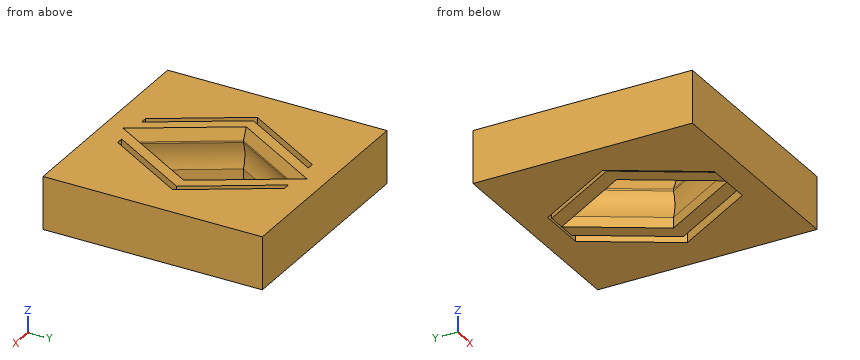
```python
from build123d import *

# Parameters (mm, degrees)
SKETCH_W      = 25
SKETCH_H      = 25
PAD_DEPTH     = 6
CHAMFER_SIZE2 = 1.3
CHAMFER_SIZE  = 0.5
POCKET_DEPTH  = 0.3


with BuildPart() as part:
    # Sketch (on XY_Plane of Origin) → Pad (new body)
    with BuildSketch(Plane.XY):
        Rectangle(SKETCH_W, SKETCH_H)
        Polygon((0, 9.5), (-5.7, 0), (0, -9.5), (5.7, 0), align=None, mode=Mode.SUBTRACT)
        Polygon((-2, 9.5), (-7.7, 0), (-2, -9.5), (-2.8, -9.5), (-8.5, 0), (-2.8, 9.5), align=None, mode=Mode.SUBTRACT)
        Polygon((2, -9.5), (7.7, 0), (2, 9.5), (2.8, 9.5), (8.5, 0), (2.8, -9.5), align=None, mode=Mode.SUBTRACT)
    extrude(amount=PAD_DEPTH)

    # Sketch002 (on Face22 of Pad) → SubtractiveLoft section 0
    with BuildSketch(Plane.XY.offset(4.5)):
        Polygon((-5.7, 0), (0, -9.5), (5.7, 0), (0, 9.5), align=None)
    # Sketch001 (on Face22 of Pad) → SubtractiveLoft section 1
    with BuildSketch(Plane.XY.offset(3)):
        Polygon((-6, 0), (0, 10), (6, 0), (0, -10), align=None)
    # Sketch003 (on Face22 of Pad) → SubtractiveLoft section 2
    with BuildSketch(Plane.XY.offset(1.5)):
        Polygon((-5.7, 0), (0, 9.5), (5.7, 0), (0, -9.5), align=None)
    loft(mode=Mode.SUBTRACT)

    # Chamfer
    chamfer_edges = [part.edges().sort_by_distance(p)[0] for p in [
        (2.85, 4.75, 6),
        (-2.85, 4.75, 6),
        (-2.85, -4.75, 6),
        (2.85, -4.75, 6),
    ]]
    chamfer_side = part.faces().sort_by_distance((-12.146447, 0, 6))[0]
    chamfer(chamfer_edges, length=CHAMFER_SIZE, length2=CHAMFER_SIZE2, reference=chamfer_side)

    # Sketch004 (on Face4 of SubtractiveLoft) → Pocket (cut)
    with BuildSketch(Plane(origin=(0, 0, 0), x_dir=(1, 0, 0), z_dir=(0, 0, -1))):
        Polygon((-8.5, 0), (-2.8, -9.5), (2.8, -9.5), (8.5, 0), (2.8, 9.5), (-2.8, 9.5), align=None)
    extrude(amount=-POCKET_DEPTH, mode=Mode.SUBTRACT)


solid = part.part
```
CAD build for the part. Positions are in the model's coordinates, mm. Round coordinates to 2 decimals unless told otherwise and drop trailing zeros. Loops run counter-clockwise (first coordinate to the right, second up) from the corner with the lowest first, then second, coordinate; pieces in that order, holes last. Notation, with made-up numbers: M 35.25,72.5 L 84.25,72.5 A10 cw 84.25,82.5 Z; hole C 60.5,-8.75 d2. An arc over 180 degrees is marked long. Return JSON: item names as keys, results as strings. Group by question number.
(1) Wall check: probe 1 along Y at (x, z) = (5.75, 4.7); probe 2 along X at (y, z) = (-6.5, 1.8); probe 3 along X at (y, z) = (-7.5, 4.45). Give the ranges that are in metal, low to high. Write a range as [from, to].
(2) Drop flat-ended pins along their axis: P1, Ø3, axis at x = 2.5, y = -2, coming from the +Z side; P2, Ø4, axis at x = 3.5, y = -2.5, coming from the -Z side. Give the stop position or say it passes through.
(3) Saw through at B-B, the plane z = 5.3. List the corners of the cut face in (x, y), and give its area (3 significant figures).
(4) Saw through at A-A, the plane y = 6. Give the number of separate pieces and of enclosed holes in the cut face, and give its area (3 significant figures).
Answer list:
{
 "1": {"probe 1": "[-12.5, -4.58], [-3.25, 3.25], [4.58, 12.5]", "probe 2": "[-12.5, -4.6], [-3.8, -1.91], [1.91, 3.8], [4.6, 12.5]", "probe 3": "[-12.5, -4], [-3.2, -1.22], [1.22, 3.2], [4, 12.5]"},
 "2": {"P1": "through", "P2": "z = 0.3"},
 "3": {"outline": "M -12.5,-12.5 L 12.5,-12.5 L 12.5,12.5 L -12.5,12.5 Z; hole M -8.5,0 L -2.8,-9.5 L -2,-9.5 L -7.7,0 L -2,9.5 L -2.8,9.5 Z; hole M -5.97,0 L 0,-9.95 L 5.97,0 L 0,9.95 Z; hole M 2,-9.5 L 2.8,-9.5 L 8.5,0 L 2.8,9.5 L 2,9.5 L 7.7,0 Z", "area": "476 mm2"},
 "4": {"separate pieces": "4", "enclosed holes": "0", "area": "112 mm2"}
}
